Part model, mm, in its own coordinate system. Coordinates: 2 decimals unless noted, no trailing zeros. Loops run counter-clockwise (first coordinate to the right, second up) from the corner with the lowest first, then second, coordinate; pieces in that order, holes last. Notation, with made-up numbers: M 46,84.25 L 57,84.25 A11 cw 57,99.25 Z; hole C 60.25,-19.75 d1. An arc over 180 degrees is marked long. Answer as a JSON object with one key per item and string values. Group by question number.
1. Drill centre lines: L1, parallel to Y at x = -34.5, z = 995; L2, parallel to Y at x = -10, z = 997.2; L3, parallel to X at y = -8.5, z = 997. Where is each one in solid material? Low to high.
2. Saw through at C-C on z = 996.15. Count the separate pieces of the cut face and the enclosed holes in it, then the cut area to 3 significant figures.
3. Saw through at A-A on x = 24. Write the cut outline in (y, z).
4. Saw through at B-B on y = 10.5. Write the cut outline in (x, z), then the cut area to 3 significant figures.
5. Drop flat-ended pins along their axis: pin 1 Ø1 at (x, z) = (4.5, 996) entering from +Y; pin 2 Ø2 at (y, z) = (-12.5, 995.5) entering from -X; pin 3 Ø0.6 at (x, z) = (-26, 996) entering from -Y. Give the stop position or say it passes through.
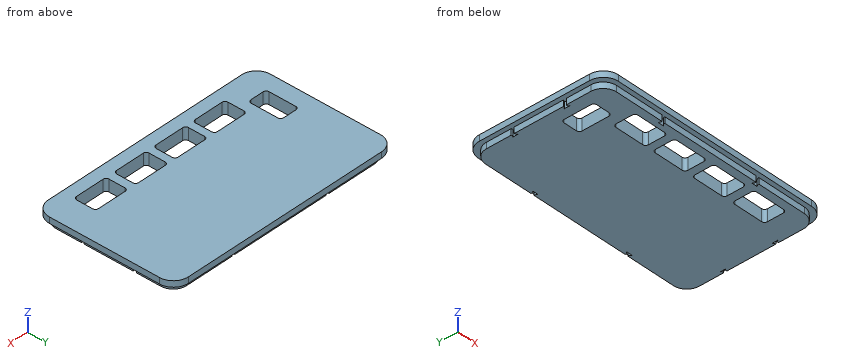
from build123d import *

# Parameters (mm, degrees)
EXTRUDE_1_DEPTH     = 2
EXTRUDE_2_DEPTH     = 2
CUT_EXTRUDE_1_DEPTH = 5


with BuildPart() as part:
    # 草图1 → 凸台-拉伸1 (new body)
    with BuildSketch(Plane.XY.offset(994.761746566)):
        with BuildLine():
            Line((-36.977217365, -23.153037779), (-20.375793692, -23.153037779))
            ThreePointArc((-20.375793692, -23.153037779), (-20.507759703, -22.594020785), (-20.875793692, -22.153037779))
            Line((-20.875793692, -22.153037779), (-18.875793692, -22.153037779))
            ThreePointArc((-18.875793692, -22.153037779), (-19.243827681, -22.594020785), (-19.375793692, -23.153037779))
            Line((-19.375793692, -23.153037779), (13.827053654, -23.153037779))
            ThreePointArc((13.827053654, -23.153037779), (13.695087643, -22.594020785), (13.327053654, -22.153037779))
            Line((13.327053654, -22.153037779), (15.327053654, -22.153037779))
            ThreePointArc((15.327053654, -22.153037779), (14.959019666, -22.594020785), (14.827053654, -23.153037779))
            Line((14.827053654, -23.153037779), (31.428477328, -23.153037779))
            ThreePointArc((31.428477328, -23.153037779), (34.610457843, -21.835018294), (35.928477328, -18.653037779))
            Line((35.928477328, -18.653037779), (35.928477328, -10.409369377))
            ThreePointArc((35.928477328, -10.409369377), (35.356461327, -10.413320038), (35.071587729, -10.909369377))
            Line((35.071587729, -10.909369377), (35.071587729, -8.909369377))
            ThreePointArc((35.071587729, -8.909369377), (35.432427989, -9.275228629), (35.928477328, -9.409369377))
            Line((35.928477328, -9.409369377), (35.928477328, 7.077967428))
            ThreePointArc((35.928477328, 7.077967428), (35.432427989, 6.943826681), (35.071587729, 6.577967428))
            Line((35.071587729, 6.577967428), (35.071587729, 8.577967428))
            ThreePointArc((35.071587729, 8.577967428), (35.356461327, 8.08191809), (35.928477328, 8.077967428))
            Line((35.928477328, 8.077967428), (35.928477328, 16.32163583))
            ThreePointArc((35.928477328, 16.32163583), (34.610457843, 19.503616346), (31.428477328, 20.82163583))
            Line((31.428477328, 20.82163583), (14.827053654, 20.82163583))
            ThreePointArc((14.827053654, 20.82163583), (14.959019666, 20.262618836), (15.327053654, 19.82163583))
            Line((15.327053654, 19.82163583), (13.327053654, 19.82163583))
            ThreePointArc((13.327053654, 19.82163583), (13.695087643, 20.262618836), (13.827053654, 20.82163583))
            Line((13.827053654, 20.82163583), (-19.375793692, 20.82163583))
            ThreePointArc((-19.375793692, 20.82163583), (-19.243827681, 20.262618836), (-18.875793692, 19.82163583))
            Line((-18.875793692, 19.82163583), (-20.875793692, 19.82163583))
            ThreePointArc((-20.875793692, 19.82163583), (-20.507759703, 20.262618836), (-20.375793692, 20.82163583))
            Line((-20.375793692, 20.82163583), (-36.977217365, 20.82163583))
            ThreePointArc((-36.977217365, 20.82163583), (-40.15919788, 19.503616346), (-41.477217365, 16.32163583))
            Line((-41.477217365, 16.32163583), (-41.477217365, 8.077967428))
            ThreePointArc((-41.477217365, 8.077967428), (-40.905201365, 8.08191809), (-40.620327767, 8.577967428))
            Line((-40.620327767, 8.577967428), (-40.620327767, 6.577967428))
            ThreePointArc((-40.620327767, 6.577967428), (-40.981168027, 6.943826681), (-41.477217365, 7.077967428))
            Line((-41.477217365, 7.077967428), (-41.477217365, -9.409369377))
            ThreePointArc((-41.477217365, -9.409369377), (-40.981168027, -9.275228629), (-40.620327767, -8.909369377))
            Line((-40.620327767, -8.909369377), (-40.620327767, -10.909369377))
            ThreePointArc((-40.620327767, -10.909369377), (-40.905201365, -10.413320038), (-41.477217365, -10.409369377))
            Line((-41.477217365, -10.409369377), (-41.477217365, -18.653037779))
            ThreePointArc((-41.477217365, -18.653037779), (-40.15919788, -21.835018294), (-36.977217365, -23.153037779))
        make_face()
    extrude(amount=EXTRUDE_1_DEPTH)

    # 草图2 → 凸台-拉伸2 (add)
    with BuildSketch(Plane.XY.offset(996.761746566)):
        with BuildLine():
            Line((-42.977217365, 17.32163583), (-42.977217365, -19.653037779))
            ThreePointArc((-42.977217365, -19.653037779), (-41.512751271, -23.188571685), (-37.977217365, -24.653037779))
            Line((-37.977217365, -24.653037779), (32.428477328, -24.653037779))
            ThreePointArc((32.428477328, -24.653037779), (35.964011233, -23.188571685), (37.428477328, -19.653037779))
            Line((37.428477328, -19.653037779), (37.428477328, 17.32163583))
            ThreePointArc((37.428477328, 17.32163583), (35.964011233, 20.857169736), (32.428477328, 22.32163583))
            Line((32.428477328, 22.32163583), (-37.977217365, 22.32163583))
            ThreePointArc((-37.977217365, 22.32163583), (-41.512751271, 20.857169736), (-42.977217365, 17.32163583))
        make_face()
    extrude(amount=EXTRUDE_2_DEPTH)

    # 草图3 → 切除-拉伸1 (cut)
    with BuildSketch(Plane.XY.offset(998.761746566)):
        with BuildLine():
            Line((-24.489796203, -20.520829455), (-18.469872403, -20.520829455))
            Line((-18.469872403, -20.520829455), (-16.599885103, -20.520829455))
            ThreePointArc((-16.599885103, -20.520829455), (-15.892778322, -20.227936236), (-15.599885103, -19.520829455))
            Line((-15.599885103, -19.520829455), (-15.599885103, -14.120887455))
            ThreePointArc((-15.599885103, -14.120887455), (-15.892778322, -13.413780673), (-16.599885103, -13.120887455))
            Line((-16.599885103, -13.120887455), (-26.359783503, -13.120887455))
            ThreePointArc((-26.359783503, -13.120887455), (-27.066890284, -13.413780673), (-27.359783503, -14.120887455))
            Line((-27.359783503, -14.120887455), (-27.359783503, -19.520829455))
            ThreePointArc((-27.359783503, -19.520829455), (-27.066890284, -20.227936236), (-26.359783503, -20.520829455))
            Line((-26.359783503, -20.520829455), (-24.489796203, -20.520829455))
        make_face()
        with BuildLine():
            Line((-10.138767501, -20.520829455), (-4.118843701, -20.520829455))
            Line((-4.118843701, -20.520829455), (-2.248856401, -20.520829455))
            ThreePointArc((-2.248856401, -20.520829455), (-1.54174962, -20.227936236), (-1.248856401, -19.520829455))
            Line((-1.248856401, -19.520829455), (-1.248856401, -14.120887455))
            ThreePointArc((-1.248856401, -14.120887455), (-1.54174962, -13.413780673), (-2.248856401, -13.120887455))
            Line((-2.248856401, -13.120887455), (-12.008754801, -13.120887455))
            ThreePointArc((-12.008754801, -13.120887455), (-12.715861582, -13.413780673), (-13.008754801, -14.120887455))
            Line((-13.008754801, -14.120887455), (-13.008754801, -19.520829455))
            ThreePointArc((-13.008754801, -19.520829455), (-12.715861582, -20.227936236), (-12.008754801, -20.520829455))
            Line((-12.008754801, -20.520829455), (-10.138767501, -20.520829455))
        make_face()
        with BuildLine():
            Line((4.212261201, -20.520829455), (10.232185001, -20.520829455))
            Line((10.232185001, -20.520829455), (12.102172301, -20.520829455))
            ThreePointArc((12.102172301, -20.520829455), (12.809279082, -20.227936236), (13.102172301, -19.520829455))
            Line((13.102172301, -19.520829455), (13.102172301, -14.120887455))
            ThreePointArc((13.102172301, -14.120887455), (12.809279082, -13.413780673), (12.102172301, -13.120887455))
            Line((12.102172301, -13.120887455), (2.342273901, -13.120887455))
            ThreePointArc((2.342273901, -13.120887455), (1.63516712, -13.413780673), (1.342273901, -14.120887455))
            Line((1.342273901, -14.120887455), (1.342273901, -19.520829455))
            ThreePointArc((1.342273901, -19.520829455), (1.63516712, -20.227936236), (2.342273901, -20.520829455))
            Line((2.342273901, -20.520829455), (4.212261201, -20.520829455))
        make_face()
        with BuildLine():
            Line((18.817290411, -20.520829455), (24.837214211, -20.520829455))
            Line((24.837214211, -20.520829455), (26.707201511, -20.520829455))
            ThreePointArc((26.707201511, -20.520829455), (27.414308292, -20.227936236), (27.707201511, -19.520829455))
            Line((27.707201511, -19.520829455), (27.707201511, -14.120887455))
            ThreePointArc((27.707201511, -14.120887455), (27.414308292, -13.413780673), (26.707201511, -13.120887455))
            Line((26.707201511, -13.120887455), (16.947303111, -13.120887455))
            ThreePointArc((16.947303111, -13.120887455), (16.24019633, -13.413780673), (15.947303111, -14.120887455))
            Line((15.947303111, -14.120887455), (15.947303111, -19.520829455))
            ThreePointArc((15.947303111, -19.520829455), (16.24019633, -20.227936236), (16.947303111, -20.520829455))
            Line((16.947303111, -20.520829455), (18.817290411, -20.520829455))
        make_face()
        with BuildLine():
            Line((-37.402959537, -5.978719817), (-37.402959537, -14.978719817))
            ThreePointArc((-37.402959537, -14.978719817), (-37.110066318, -15.685826598), (-36.402959537, -15.978719817))
            Line((-36.402959537, -15.978719817), (-31.902959537, -15.978719817))
            ThreePointArc((-31.902959537, -15.978719817), (-31.195852756, -15.685826598), (-30.902959537, -14.978719817))
            Line((-30.902959537, -14.978719817), (-30.902959537, -5.978719817))
            ThreePointArc((-30.902959537, -5.978719817), (-31.195852756, -5.271613035), (-31.902959537, -4.978719817))
            Line((-31.902959537, -4.978719817), (-36.402959537, -4.978719817))
            ThreePointArc((-36.402959537, -4.978719817), (-37.110066318, -5.271613035), (-37.402959537, -5.978719817))
        make_face()
    extrude(amount=-CUT_EXTRUDE_1_DEPTH, mode=Mode.SUBTRACT)


solid = part.part
Outcome:
{
 "1": {"L1": "y = -23.15 to -15.98, -4.98 to 20.82", "L2": "y = -24.65 to -20.52, -13.12 to 22.32", "L3": "x = -42.98 to -37.4, -30.9 to 37.43"},
 "2": {"separate pieces": "1", "enclosed holes": "5", "area": "2,960 mm²"},
 "3": {"outline": "M -24.65,996.76 L -23.15,996.76 L -23.15,994.76 L -20.52,994.76 L -20.52,998.76 L -24.65,998.76 Z; M -13.12,994.76 L 20.82,994.76 L 20.82,996.76 L 22.32,996.76 L 22.32,998.76 L -13.12,998.76 Z"},
 "4": {"outline": "M -42.98,996.76 L -41.48,996.76 L -41.48,994.76 L 35.93,994.76 L 35.93,996.76 L 37.43,996.76 L 37.43,998.76 L -42.98,998.76 Z", "area": "316 mm²"},
 "5": {"pin 1": "stops at y = 20.82", "pin 2": "stops at x = -41.48", "pin 3": "stops at y = -23.15"}
}
